```python
from build123d import *

# Parameters (mm, degrees)
SKETCH_1_R          = 8.5
SKETCH_1_R_2        = 4.5
EXTRUDE_1_DEPTH     = 15
SKETCH_2_W          = 30
SKETCH_2_H          = 60
CUT_EXTRUDE_1_DEPTH = 5
SKETCH_3_R          = 3
EXTRUDE_2_DEPTH     = 4


with BuildPart() as part:
    # Эскиз1 → Бобышка-Вытянуть1 (new, symmetric)
    with BuildSketch(Plane.XY):
        with BuildLine():
            ThreePointArc((12.459935794, -1), (0, 12.5), (-12.459935794, -1))
            Line((-12.459935794, -1), (-8.47275634, -50.68))
            ThreePointArc((-8.47275634, -50.68), (0, -58.5), (8.47275634, -50.68))
            Line((8.47275634, -50.68), (12.459935794, -1))
        make_face()
        Circle(SKETCH_1_R, mode=Mode.SUBTRACT)
        with Locations((0, -50)):
            Circle(SKETCH_1_R_2, mode=Mode.SUBTRACT)
    extrude(amount=EXTRUDE_1_DEPTH, both=True)

    # Эскиз2 → Вырез-Вытянуть1 (cut, symmetric)
    with BuildSketch(Plane.XY):
        with Locations((0, -50)):
            Rectangle(SKETCH_2_W, SKETCH_2_H)
    extrude(amount=CUT_EXTRUDE_1_DEPTH, both=True, mode=Mode.SUBTRACT)

    # Эскиз3 → Бобышка-Вытянуть2 (add, symmetric)
    with BuildSketch(Plane.XY):
        with BuildLine():
            Line((-31.819805153, 24.748737342), (-11.636459779, 4.565391967))
            ThreePointArc((-11.636459779, 4.565391967), (-8.838834765, 8.838834765), (-4.565391967, 11.636459779))
            Line((-4.565391967, 11.636459779), (-24.748737342, 31.819805153))
            ThreePointArc((-24.748737342, 31.819805153), (-31.819805153, 31.819805153), (-31.819805153, 24.748737342))
        make_face()
        with Locations((-28.284271247, 28.284271247)):
            Circle(SKETCH_3_R, mode=Mode.SUBTRACT)
    extrude(amount=EXTRUDE_2_DEPTH, both=True)


solid = part.part
```
Could you check a few things on this model? Use its own coordinates, in mm. A direction names the side the tool comes from. Coordinates: 2 decimals unless noted, no trailing zeros. Write each loop counter-clockwise with the first axis right and the second up, starting at its lowest first coordinate (ties: lowest second). Pieces come first, ordered by that corner, then holes. Notation, with made-up numbers: (-6, 45.5) -> (15, 45.5) arc R17 cw to (15, 67.5) -> close; hole circle Ø11 at (74, 46). An arc over 180 degrees is marked (long way). Write item = value, one per line. Start each with the question number.
(1) Will these pins go through, and if not, where does the flat tip stop? pin 1 (5 mm diameter, centred on y = -38.5, z = -8, fed in from +X); pin 2 (5 mm diameter, centred on y = -24.5, z = 5, fed in from +X); pin 3 (8 mm diameter, centred on x = 0, y = -50, fed in from -Z); pin 4 (3 mm diameter, centred on x = 2.5, z = 1.5, fed in from -Y).
(2) I want a section at C-C (z = 6.25). Please give me the cut outline in (x, y).
(3) I want a section at A-A (x = 0). Please give me the cut outline in (y, z), plus the area to 4 significant figures.
(4) I want a section at D-D (z = 2). Please give me the cut outline in (x, y), plus the area to 3 significant figures.
(5) I want a section at B-B (y = 0). Please give me the cut outline in (x, z), plus the area to 3 significant figures.
(6) We'd pull the mould along X, two halves only. Please class faces 1 (the face through (-0.18, -58.5, -9.93)), 2 (the face through (-0.98, -54.39, -10.07)), 3 (the face through (0, -35, -5)), 4 (the face through (-25.51, 27.14, -0.06)): released by +X, released by -X, zero draft, split by the parting line, or undercut.
(7) I need wall thicknesses on line 1 (Y direction, x = 0, z = -4.75); line 2 (Y direction, x = 2, z = 5.25); line 3 (Y direction, x = -3.5, z = 9.5). Which ranges of each line are inside material? Lowest first, please. Write a range as [from, to].
(8) Which directions (+Z, -Z, +X, -X, +Y, -Y) give clear straight access to the entire face, cutting with the end or side of a thin tool? Please do faces 5 (the face through (-19, 19, 4)), 6 (the face through (-19, 19, -4)), 7 (the face through (0, -20, 0)).
Result set:
q1.pin_1 = 9.65
q1.pin_2 = 10.77
q1.pin_3 = through
q1.pin_4 = -20
q2.outline = (-12.46, -1) -> (-8.47, -50.68) arc R8.5 ccw to (8.47, -50.68) -> (12.46, -1) arc R12.5 ccw (long way) to start; hole circle Ø17 at (0, 0); hole circle Ø9 at (0, -50)
q3.outline = (-58.5, -15) -> (-54.5, -15) -> (-54.5, -5) -> (-58.5, -5) -> close; (-58.5, 5) -> (-54.5, 5) -> (-54.5, 15) -> (-58.5, 15) -> close; (-45.5, -15) -> (-8.5, -15) -> (-8.5, 15) -> (-45.5, 15) -> (-45.5, 5) -> (-20, 5) -> (-20, -5) -> (-45.5, -5) -> close; (8.5, -15) -> (12.5, -15) -> (12.5, 15) -> (8.5, 15) -> close
q3.area = 1,055 mm2
q4.outline = (-31.82, 24.75) -> (-11.64, 4.57) arc R12.5 ccw to (-12.46, -1) -> (-10.94, -20) -> (10.94, -20) -> (12.46, -1) arc R12.5 ccw to (-4.57, 11.64) -> (-24.75, 31.82) arc R5 ccw to start; hole circle Ø6 at (-28.28, 28.28); hole circle Ø17 at (0, 0)
q4.area = 777 mm2
q5.outline = (-12.5, -15) -> (-8.5, -15) -> (-8.5, 15) -> (-12.5, 15) -> close; (8.5, -15) -> (12.5, -15) -> (12.5, 15) -> (8.5, 15) -> close
q5.area = 240 mm2
q6.face_1 = split by the parting line
q6.face_2 = undercut
q6.face_3 = zero draft
q6.face_4 = undercut
q7.line_1 = [-20, -8.5], [8.5, 12.5]
q7.line_2 = [-58.26, -54.03], [-45.97, -8.26], [8.26, 12.34]
q7.line_3 = [-57.75, -52.83], [-47.17, -7.75], [7.75, 12]
q8.face_5 = +Z, -X, +Y
q8.face_6 = -Z, -X, +Y
q8.face_7 = +X, -X, -Y
